Here's how the part is built. I have some questions about the finished solid (model axes, mm). A direction names the side the tool comes from. Give positions to 0.01 mm unless a question says otherwise; leave off trailing zeros. Write each loop counter-clockwise with the first axis right and the second up, starting at its lowest first coordinate (ties: lowest second). Pieces come first, ordered by that corner, then holes. Notation, with made-up numbers: M 43,86 L 95,86 A18 cw 95,96 Z; hole C 61.25,36 d11. An arc over 180 degrees is marked long. Answer as CSV lines item,"result". Start each with the question number.
Q1. For pin 1 (5 mm diameter, centred on x = -59.5, z = 69.5, fed in from -Y); pin 2 (8 mm diameter, centred on y = -26, z = 35.5, fed in from -X); pin 3 (8 mm diameter, centred on x = -56, z = 70, fed in from +Y), each with a flat end and sliding along its axis, tell me the tip position at first contact or that it passes through.
Q2. If I drill on line 1 along Y through (x, z) = (-26, 30); line 2 along X through (y, z) = (-27, 42); line 3 along Y through (x, z) = (-32.5, 28.5), over which ranges is the centre line in solid material (lowest first)?
Q3. Suppose I cut it at A-A (y = -0.5). Write out the boundary of the cut face in (x, z), then the cut area to 3 significant figures.
Q4. On a 3-axis mill with a long thin cutter (end or side, diameter ignored), from which of +Z, -Z, +X, -X, +Y, -Y can I reach the whole of each face in a straight line? I mean faces 4 (the flat face through (56, 12.7, 72)), 5 (the flat face through (-1, 38.1, 25)), 6 (the flat face through (-1, -38.1, 25)), 7 (the flat face through (0, 29.21, 39)). Say none if no direction works.
Q5. Thinking about a two-plate mould opening in X: for faces 1 (the flat face through (57.24, -0.18, 70.55)), 2 (the flat face through (0, -29.21, 39)), 3 (the flat face through (-56, -12.7, 72)), which applies, +X half, -X half, draft (parallel to the pull), parting line (faces both ways), or undercut?
Q6. Suppose I cut it at B-B (x = -11.5). Write out the boundary of the cut face in (y, z), then the cut area to 3 significant figures.
Q7. Suppose I cut it at D-D (x = -45). Write out the boundary of the cut face in (y, z), then the cut area to 3 significant figures.
Q8. Suppose I cut it at C-C (z = 28). Write out the boundary of the cut face in (x, y), then the cut area to 3 significant figures.
```python
from build123d import *

# Parameters (mm, degrees)
F0_W      = 101.6
F0_H      = 76.2
F1_DEPTH  = 76.2
F2_W      = 58.42
F2_H      = 58.42
F3_DEPTH  = 228.6
F4_W      = 101.6
F4_H      = 25.4
F5_DEPTH  = 25.4
F6_W      = 101.6
F6_H      = 25.4
F7_DEPTH  = 25.4
F9_DEPTH  = 228.6
F10_W     = 25.4
F10_H     = 10.16
F11_DEPTH = 12.7
F13_DEPTH = 228.6
F14_W     = 25.4
F14_H     = 10.16
F15_DEPTH = 12.7
F17_DEPTH = 228.6


with BuildPart() as f1:
    # F0 (on Top) → F1 (new body)
    with BuildSketch(Plane.XY):
        Rectangle(F0_W, F0_H)
    extrude(amount=F1_DEPTH)

    # F2 (on face) → F3 (cut)
    with BuildSketch(Plane.XY.offset(76.2)):
        Rectangle(F2_W, F2_H)
    extrude(amount=-F3_DEPTH, mode=Mode.SUBTRACT)

    # F4 (on face) → F5 (join)
    with BuildSketch(Plane(origin=(0, 38.1, 0), x_dir=(-1, 0, 0), z_dir=(0, 1, 0))):
        with Locations((0, 63.5)):
            Rectangle(F4_W, F4_H)
    extrude(amount=F5_DEPTH)

    # F6 (on face) → F7 (join)
    with BuildSketch(Plane.XZ.offset(38.1)):
        with Locations((0, 63.5)):
            Rectangle(F6_W, F6_H)
    extrude(amount=F7_DEPTH)

    # F8 (on face) → F9 (cut)
    with BuildSketch(Plane.YZ.offset(50.8)):
        Polygon((-38.1, 50.8), (-63.5, 73.66), (-63.5, 50.8), align=None)
        Polygon((63.5, 50.8), (63.5, 73.66), (38.1, 50.8), align=None)
    extrude(amount=-F9_DEPTH, mode=Mode.SUBTRACT)

    # F10 (on face) → F11 (join)
    with BuildSketch(Plane.YZ.offset(50.8)):
        with Locations((0, 71.12)):
            Rectangle(F10_W, F10_H)
    extrude(amount=F11_DEPTH)

    # F12 (on face) → F13 (cut)
    with BuildSketch(Plane.XZ.offset(12.7)):
        Polygon((63.5, 66.04), (63.5, 74.93), (50.8, 66.04), align=None)
    extrude(amount=-F13_DEPTH, mode=Mode.SUBTRACT)

    # F14 (on face) → F15 (join)
    with BuildSketch(Plane(origin=(-50.8, 0, 0), x_dir=(0, -1, 0), z_dir=(-1, 0, 0))):
        with Locations((0, 71.12)):
            Rectangle(F14_W, F14_H)
    extrude(amount=F15_DEPTH)

    # F16 (on face) → F17 (cut)
    with BuildSketch(Plane(origin=(0, 12.7, 0), x_dir=(-1, 0, 0), z_dir=(0, 1, 0))):
        Polygon((63.5, 66.04), (63.5, 74.93), (50.8, 66.04), align=None)
    extrude(amount=-F17_DEPTH, mode=Mode.SUBTRACT)


solid = f1.part
```
Resolved:
1,pin 1,"y = -12.7"
1,pin 2,"x = -50.8"
1,pin 3,"y = 12.7"
2,line 1,"-38.1 to -29.21, 29.21 to 38.1"
2,line 2,"-50.8 to -29.21, 29.21 to 50.8"
2,line 3,"-38.1 to 38.1"
3,outline,"M -63.5,74.93 L -50.8,66.04 L -50.8,0 L -29.21,0 L -29.21,76.2 L -63.5,76.2 Z; M 29.21,0 L 50.8,0 L 50.8,66.04 L 63.5,74.93 L 63.5,76.2 L 29.21,76.2 Z"
3,area,"3,440 mm^2"
4,face 4,"+Z, -Z, +X, +Y"
4,face 5,"-Z, +X, -X, +Y"
4,face 6,"-Z, +X, -X, -Y"
4,face 7,"+Z, -Z"
5,face 1,"+X half"
5,face 2,"undercut"
5,face 3,"draft"
6,outline,"M -63.5,73.66 L -38.1,50.8 L -38.1,0 L -29.21,0 L -29.21,76.2 L -63.5,76.2 Z; M 29.21,0 L 38.1,0 L 38.1,50.8 L 63.5,73.66 L 63.5,76.2 L 29.21,76.2 Z"
6,area,"2,060 mm^2"
7,outline,"M -63.5,73.66 L -38.1,50.8 L -38.1,0 L 38.1,0 L 38.1,50.8 L 63.5,73.66 L 63.5,76.2 L -63.5,76.2 Z"
7,area,"6,520 mm^2"
8,outline,"M -50.8,-38.1 L 50.8,-38.1 L 50.8,38.1 L -50.8,38.1 Z; hole M -29.21,-29.21 L 29.21,-29.21 L 29.21,29.21 L -29.21,29.21 Z"
8,area,"4,330 mm^2"
